Build history of the part. All positions in model axes, mm. Face numbers are marked on the shaded views. A direction names the side the tool comes from. Coordinates: 2 decimals unless noted, no trailing zeros. Order: outer loops, then holes, each group sorted by start corner. A loop starts at its lowest first (then second) coordinate and runs counter-clockwise, first axis right, second up. Notation, with made-up numbers: (4, -25) - (39, -25) arc R16 cw to (39, 2) - close; hole circle Ø2 at (-17.75, -6.5). An arc over 180 degrees is marked (long way). Return JSON: item names as keys, results as strings.
Autodesk Inventor part; units mm, degrees
ref_plane "YZ Plane" through (0, 0, 0) normal (1, 0, 0) x (0, 1, 0)
ref_plane "XZ Plane" through (0, 0, 0) normal (0, 1, 0) x (-1, 0, 0)
ref_plane "XY Plane" through (0, 0, 0) normal (0, 0, 1) x (1, 0, 0)
sketch "Эскиз1" plane through (0, 0, 0) normal (0, 1, 0) x (-1, 0, 0)
  line L0 (0, 0) -> (20, 0)
  line L1 (20, 0) -> (20, -20)
  line L2 (20, -20) -> (0, -20)
  line L3 (0, -20) -> (0, 0)
  line L4 (20, 0) -> (20, -2)
  line L5 (0, -20) -> (2, -20)
  line L6 (20, -2) -> (2, -20)
  dimension "d0" = 20
  dimension "d1" = 20
  dimension "d2" = 2
  dimension "d3" = 2
extrude "Выдавливание1" add sketch "Эскиз1" along normal blind 17 contours L0 L1 L6 L2 L3
sketch "Эскиз2" plane through (0, 0, -20) normal (0, 0, -1) x (-1, 0, 0)
  line L0 (0, 17) -> (2, 17)
  line L1 (2, 17) -> (2, 15)
  line L2 (2, 0) -> (2, 17)
  line L3 (2, 15) -> (20, 15)
  line L4 (20, 0) -> (20, 17)
  line L5 (0, 0) -> (2, 0)
  line L6 (2, 0) -> (2, 2)
  line L7 (2, 2) -> (20, 2)
  line L8 (20, 2) -> (20, 15)
  line L9 (2, 15) -> (2, 2)
  dimension "d6" = 2
  dimension "d7" = 2
extrude "Выдавливание2" cut sketch "Эскиз2" against normal blind 18
sketch "Эскиз3" plane through (0, 0, -2) normal (0, 0, -1) x (-1, 0, 0)
  line L0 (0, 0) -> (0, 17)
  line L1 (10, 10.2321) -> (10, 10.5)
  line L2 (10, 10.5) -> (11, 10.5)
  line L3 (11, 6.5) -> (9, 6.5)
  line L4 (9, 10.5) -> (10, 10.5)
  arc A0 (11, 6.5) -> (11, 10.5) centre (11, 8.5) ccw
  arc A1 (9, 10.5) -> (9, 6.5) centre (9, 8.5) ccw
  line L5 (10, 10.5) -> (10, 8.5)
  line L6 (0, 8.5) -> (7, 8.5)
  line L7 (9, 8.5) -> (10, 8.5)
  dimension "d10" = 10
  dimension "d11" = 2
  dimension "d13" = 1
extrude "Выдавливание3" cut sketch "Эскиз3" against normal blind 10
sketch "Эскиз4" plane through (-2, 2, -20) normal (-1, 0, 0) x (0, 0, 1)
  line L0 (0, 0) -> (0, 13)
  line L1 (0, 6.5) -> (10, 6.5)
  line L2 (10, 8.2321) -> (10, 8.5)
  line L3 (10, 8.5) -> (9, 8.5)
  line L4 (9, 4.5) -> (11, 4.5)
  line L5 (11, 8.5) -> (10, 8.5)
  arc A0 (9, 8.5) -> (9, 4.5) centre (9, 6.5) ccw
  arc A1 (11, 4.5) -> (11, 8.5) centre (11, 6.5) ccw
  point P0 (20, -2)
  dimension "d17" = 10
extrude "Выдавливание4" cut sketch "Эскиз4" against normal blind 2
properties part number "угол"
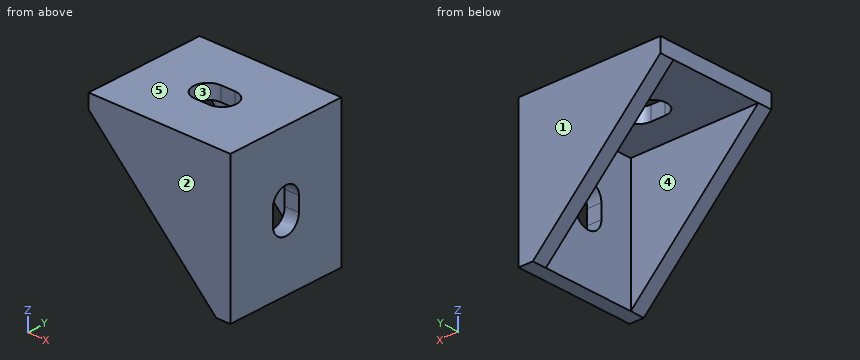
1. Tool access for the marked faces 4 and 5: list every direction of +Z, -Z, +X, -X, +Y, -Y with a clear straight run to the whole face (end or side of a thin tool).
Check values:
{"face 4": "-Z, -X", "face 5": "+Z, +X, -X, +Y, -Y"}
2. Probe L1, parallel to Y at x = -3.25, z = -13; L2, parallel to Z at x = -18.75, y = 8. List the from-to ranges inside material, lowest first.
Check values:
{"L1": "0 to 2, 15 to 17", "L2": "-2 to 0"}
3. Cut at C-C on y = 8.75. Give the cut face in (x, z).
Check values:
{"outline": "(-20, -2) - (-12.98, -2) - (-12.98, 0) - (-20, 0) - close; (-7.02, -2) - (-2, -2) - (-2, -7.02) - (0, -7.02) - (0, 0) - (-7.02, 0) - close; (-2, -20) - (0, -20) - (0, -12.98) - (-2, -12.98) - close"}
4. Cut at B-B on x = -14.75. Give the cut face in (y, z), plus the area to 3 significant figures.
Check values:
{"outline": "(0, -7.25) - (2, -7.25) - (2, -2) - (15, -2) - (15, -7.25) - (17, -7.25) - (17, 0) - (0, 0) - close", "area": "55.0 mm²"}
5. Drop flat-ended pins along their axis: pin 1 (10 mm diameter, centred on x = -8.5, y = 12.5, fed in from +Z); pin 2 (6.5 mm diameter, centred on y = 8, z = -11, fed in from -X); pin 3 (1 mm diameter, centred on y = 7.5, z = -11.5, fed in from -X); pin 4 (10 mm diameter, centred on x = -17.5, y = 14.5, fed in from -Z). Give the stop position or say it passes through.
Check values:
{"pin 1": "z = 0", "pin 2": "x = -2", "pin 3": "through", "pin 4": "z = -9.47"}
6. Cut at D-D on z = -4.25. Give the cut face in (x, y), plus the area to 3 significant figures.
Check values:
{"outline": "(-17.75, 0) - (0, 0) - (0, 17) - (-17.75, 17) - (-17.75, 15) - (-2, 15) - (-2, 2) - (-17.75, 2) - close", "area": "97.0 mm²"}
7. Cut at A-A on z = -9.75. Give the cut face in (x, y), plus the area to 3 significant figures.
Check values:
{"outline": "(-12.25, 0) - (0, 0) - (0, 6.5) - (-2, 6.5) - (-2, 2) - (-12.25, 2) - close; (-12.25, 15) - (-2, 15) - (-2, 10.5) - (0, 10.5) - (0, 17) - (-12.25, 17) - close", "area": "67.0 mm²"}
8. Mould opens along Y. For the marked faces 1, 2 and 3 say: pulls with the +Y half, pulls with the -Y half, needs draft (parallel to the pull), parting line crosses it, or undercut.
Check values:
{"face 1": "pulls with the +Y half", "face 2": "pulls with the -Y half", "face 3": "undercut"}
